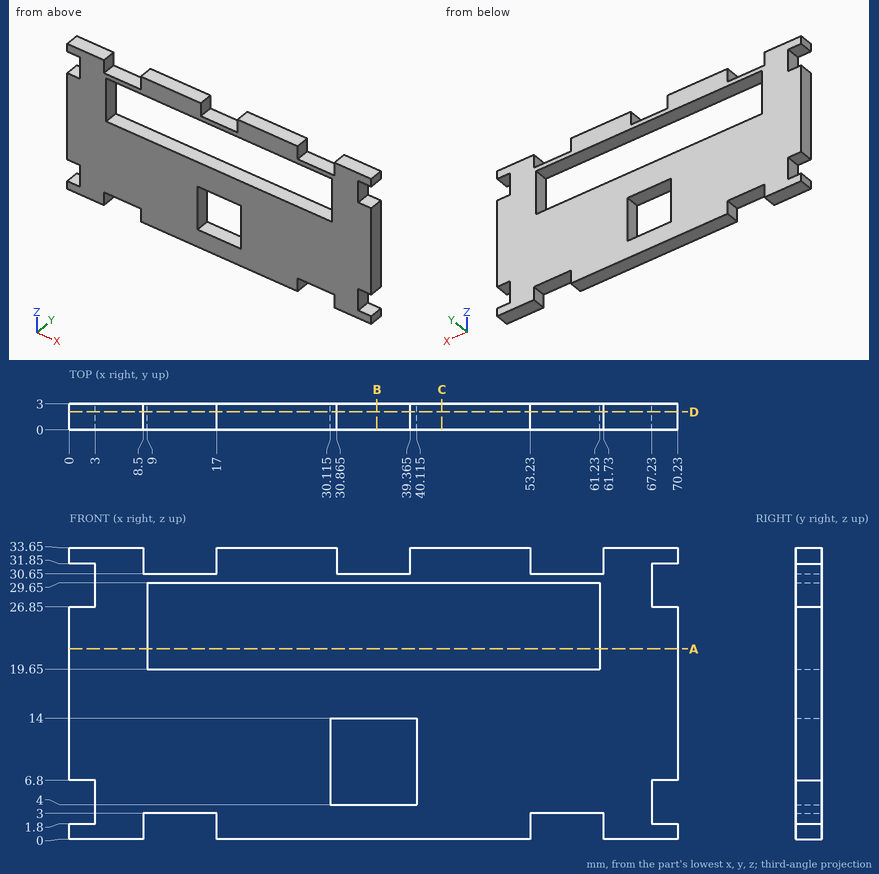
Geometry: see drawing. Coordinates: mm, zero at the bounding-box minimum. Give positions to 0.01 mm unless a question says otherwise; leave off trailing zeros. Loops run counter-clockwise (first coordinate to the right, second up) from the corner with the lowest first, then second, coordinate; pieces in that order, holes last. Notation, with made-up numbers: (59.25, -5) - (87.25, -5) arc R25 ccw to (87.25, 19) - close; hole circle Ø10 at (15, 48.25). An arc over 180 degrees is marked (long way). Answer as CSV lines item,"result". Start each with the question number.
1. Ray query, L1, parallel to X at y = 1.75, z = 2; L2, parallel to X at y = 1.7, z = 31.5 (3 decimals); L3, parallel to X at y = 0.4, z = 29. Return the intervals inside material, ascending.
2. Section A-A, the plane z = 22. Return loops of the section in (x, y).
3. Section C-C, the plane x = 43. Return loops of the section in (y, z).
4. Section D-D, the plane y = 2.1. Give the number of separate pieces and of enclosed holes in the cut face, plus the area to 3 significant figures.
5. Section B-B, the plane x = 35.5. Return loops of the section in (y, z), plus the area to 4 significant figures.
6. Pin query (flat end, axial travel): P1, Ø0.9, axis at x = 13, y = 1, coming from the +Z side; P2, Ø2, axis at x = 18.5, z = 22, coming from the +Y side; P3, Ø0.9, axis at y = 1.5, z = 29.5, coming from the -X side. Return the tip coordinate at first contact, or that it passes through.
Answers:
1,L1,"x = 3 to 8.5, 17 to 53.23, 61.73 to 67.23"
1,L2,"x = 3 to 8.5, 17 to 30.865, 39.365 to 53.23, 61.73 to 67.23"
1,L3,"x = 3 to 9, 61.23 to 67.23"
2,outline,"(0, 0) - (9, 0) - (9, 3) - (0, 3) - close; (61.23, 0) - (70.23, 0) - (70.23, 3) - (61.23, 3) - close"
3,outline,"(0, 0) - (3, 0) - (3, 19.65) - (0, 19.65) - close; (0, 29.65) - (3, 29.65) - (3, 33.65) - (0, 33.65) - close"
4,separate pieces,"1"
4,enclosed holes,"2"
4,area,"1,550 mm2"
5,outline,"(0, 0) - (3, 0) - (3, 4) - (0, 4) - close; (0, 14) - (3, 14) - (3, 19.65) - (0, 19.65) - close; (0, 29.65) - (3, 29.65) - (3, 30.65) - (0, 30.65) - close"
5,area,"31.95 mm2"
6,P1,"stops at z = 30.65"
6,P2,"passes through"
6,P3,"stops at x = 3"
